Read the model definition and answer for the solid it produces. Units are mm, in the model's axes. Face numbers are marked on the shaded views. Round coordinates to 2 decimals unless told otherwise and drop trailing zeros. Write each question's results on one line, items separated by ' | '.
Autodesk Inventor part; units mm, degrees
ref_plane "Work Plane1" through (10, 0, 0) normal (1, 0, 0) x (0, 1, 0)
ref_plane "XZ Plane" through (0, 0, 0) normal (0, 1, 0) x (-1, 0, 0)
ref_plane "XY Plane" through (0, 0, 0) normal (0, 0, 1) x (1, 0, 0)
sketch "Sketch2" plane through (0, 0, 0) normal (0, 0, 1) x (1, 0, 0)
  line L0 (0, 0) -> (20, 0)
  line L1 (20, 0) -> (20, 7)
  line L2 (20, 7) -> (0, 7)
  line L3 (0, 7) -> (0, 0)
  dimension "d0" = 20
  dimension "d1" = 7
extrude "Extrusion1" add sketch "Sketch2" along normal blind 40
ref_plane "Work Plane1" through (10, 0, 0) normal (1, 0, 0) x (0, 1, 0)
sketch "Sketch3" plane through (10, 0, 0) normal (1, 0, 0) x (0, 1, 0)
  line L0 (7, 40) -> (0, 40) construction
  line L1 (0, 40) -> (0, 30) construction
  line L2 (0, 0) -> (0, 40) construction
  line L3 (0, 30) -> (2, 30) construction
  line L4 (0, 30) -> (0, 23)
  line L5 (0, 23) -> (0.5, 23)
  line L6 (0, 30) -> (2, 30)
  arc A0 (0.5, 23) -> (1.333, 26.4822) centre (-72.4911, 42.3017) ccw
  line L7 (2, 30) -> (2, 26.4822)
  line L8 (2, 26.4822) -> (1.333, 26.4822)
  dimension "d4" = 10
  dimension "d5" = 2
  dimension "d6" = 7
  dimension "d9" = 0.5
  dimension "d10" = 75.5
revolve "Revolution1" cut sketch "Sketch3" angle 360 about axis through (10, 0, 30) along (0, 1, 0)
sketch "Sketch5" plane through (10, 2, 30) normal (0, -1, 0) x (1, 0, 0)
  circle A0 centre (0, 0) radius 3.5178
  circle A1 centre (0, 2) radius 1
  circle A2 centre (0, -2) radius 1
  line L0 (1.4669, 0) -> (-1.3764, 0) construction
  point P0 (-10, -30)
  dimension "d11" = 2
  dimension "d12" = 2
  dimension "d13" = 2
  dimension "d14" = 2
hole "Hole1" at (10, 2, 32) direction (0, 1, 0) diameter 2 depth 10 countersink diameter 2.5 countersink angle 60
sketch "Sketch6" plane through (10, 2, 30) normal (0, -1, 0) x (1, 0, 0)
  line L0 (0, 0) -> (1.9071, 0) construction
  circle A0 centre (0, -2) radius 1
  point P0 (-10, -30)
  dimension "d22" = 2
  dimension "d23" = 2
extrude "Extrusion2" cut sketch "Sketch6" against normal blind 40
sketch "Sketch7" plane through (10, 0, 0) normal (1, 0, 0) x (0, 1, 0)
  line L0 (2, 27) -> (2, 29) construction
  line L1 (2, 28) -> (3.2187, 28) construction
  line L2 (2.5, 26.7113) -> (2, 27)
  line L3 (2, 27) -> (2, 29) construction
  line L4 (2, 27) -> (2.7064, 27) construction
  line L5 (2, 29) -> (2.7329, 29) construction
  line L6 (2, 29) -> (7, 29)
  line L7 (2, 28) -> (2, 27)
  line L8 (2.5, 26.7113) -> (7.9836, 26.7113)
  line L9 (2, 28) -> (7.9836, 28)
  line L10 (8.4909, 28) -> (8.4909, 26.7113)
  line L11 (8.4909, 26.7113) -> (7.9836, 26.7113)
  line L12 (7.9836, 28) -> (8.4909, 28)
  point P0 (0, 0)
  point P1 (2.5, 28)
  dimension "d26" = 30
revolve "Revolution2" cut sketch "Sketch7" angle 360 about axis through (10, 2, 28) along (0, 1, 0)
fillet "Fillet1" radius 2 2 edges at (0, 3.5, 0) (20, 3.5, 0)
sketch "Sketch9" plane through (0, 7, 40) normal (0, 1, 0) x (1, 0, 0)
  circle A0 centre (2, 2) radius 0.75
  circle A1 centre (2, 21) radius 0.75
  circle A2 centre (2, 31) radius 0.75
  circle A3 centre (2, 38) radius 0.75
  circle A4 centre (18, 38) radius 0.75
  circle A5 centre (18, 31) radius 0.75
  circle A6 centre (18, 21) radius 0.75
  circle A7 centre (10, 21) radius 0.75
  point P0 (0, 40)
  point P1 (18, 2)
hole "Hole3" at (2, 7, 38) at (2, 7, 19) at (2, 7, 9) at (2, 7, 2) at (18, 7, 2) at (18, 7, 9) at (18, 7, 19) at (10, 7, 19) at (18, 7, 38) direction (0, -1, 0) diameter 1.5 depth 10 counterbore diameter 3 counterbore depth 2
properties part number "Nắp hộp piston" material "Iron, Gray"
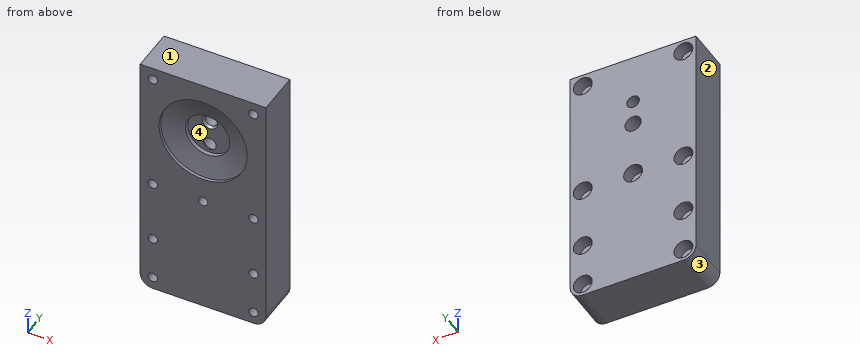
1. Given P1, Ø2.5, axis at x = 18, z = 19, coming from the +Y side; P2, Ø1.8, axis at x = 10, z = 32, coming from the +Y side; P3, Ø2.5, axis at x = 10, z = 28, coming from the -Y side, each flat-ended and moving along its own axis, determine where each tip first touches the part or whether it passes through.
Completed:
P1: stops at y = 5 | P2: passes through | P3: stops at y = 2
2. Determine the mould class of the marked faces 1, 2, 3 and 4 for opening direction Z: released by +Z, released by -Z, zero draft, split by the parting line, or undercut.
Completed:
face 1: released by +Z | face 2: zero draft | face 3: released by -Z | face 4: undercut
3. Find section A-A, the plane y = 3. Count the separate pieces of the cut face and the enclosed holes in it, then the cut area to 3 significant figures.
Completed:
separate pieces: 1 | enclosed holes: 11 | area: 774 mm2
4. Find the intervals of material crossed by L1, parallel to X at y = 2.45, z = 19; L2, parallel to X at y = 1.85, z = 38; L3, parallel to Z at x = 10, y = 5.2, in increasing order.
Completed:
L1: x = 0 to 1.25, 2.75 to 9.25, 10.75 to 17.25, 18.75 to 20 | L2: x = 0 to 1.25, 2.75 to 17.25, 18.75 to 20 | L3: z = 0 to 17.5, 20.5 to 26.71, 29.29 to 31, 33 to 40
